The model under review builds one solid part; all positions refer to its coordinate system, in mm. Face numbers are marked on the shaded views. A direction names the side the tool comes from. Round coordinates to 2 decimals unless told otherwise and drop trailing zeros. Write each loop counter-clockwise with the first axis right and the second up, starting at its lowest first coordinate (ties: lowest second). Pieces come first, ordered by that corner, then holes. Notation, with made-up numbers: M 38,18.25 L 77,18.25 A18 cw 77,34.25 Z; hole C 28.25,-7 d2. An arc over 180 degrees is marked long. One line per item, written item: value. Start each with the question number.
1) Wall thickness on probe 1 along Y at (x, z) = (1.25, 19.5); probe 2 along Y at (x, z) = (3.5, 24); probe 3 along Z at (x, y) = (4.75, 10.5): over which ranges is each line inside the solid? List them lowest first.
2) Mouldability with a two-part tool opening along Z and no side actions: class the marked faces 1, 2 and 3 as +Z half, -Z half, draft (parallel to the pull), parting line (faces both ways), or undercut.
3) Take a section at A-A, the plane x = 5.75. Write out the cut boundary in (y, z), and give its area (3 significant figures).
4) Take a section at C-C, the plane z = 13.75. Write out the cut boundary in (x, y), and give its area (3 significant figures).
5) Tool access review of the marked faces 4, 5 and 6: name each direction out of +Z, -Z, +X, -X, +Y, -Y from which nothing blocks a thin tool from reaching the whole face with its end or side.
6) For P1, Ø1.5, axis at y = 17.5, z = 5, coming from the -X side, flat-tipped, find the tip position at first contact; note if it passes through.
7) Take a section at B-B, the plane y = 12.7. Write out the cut boundary in (x, z).
from build123d import *

# Parameters (mm, degrees)
F0_W     = 25.4
F0_H     = 25.4
F1_DEPTH = 6.35
F2_R     = 2.54
F3_DEPTH = 6.35
F4_R     = 2.54
F5_DEPTH = 6.35


with BuildPart() as f1:
    # F0 (on Right) → F1 (new body)
    with BuildSketch(Plane.YZ):
        with Locations((12.7, 12.7)):
            Rectangle(F0_W, F0_H)
    extrude(amount=F1_DEPTH)

    # F2 (on face) → F3 (cut)
    with BuildSketch(Plane.YZ.offset(6.35)):
        with Locations((12.7, 0)):
            Circle(F2_R)
        with Locations((0, 12.7)):
            Circle(F2_R)
        with Locations((12.7, 25.4)):
            Circle(F2_R)
    extrude(amount=-F3_DEPTH, mode=Mode.SUBTRACT)

    # F4 (on face) → F5 (join)
    with BuildSketch(Plane.YZ.offset(6.35)):
        with Locations((25.4, 12.7)):
            Circle(F4_R)
    extrude(amount=-F5_DEPTH)


solid = f1.part
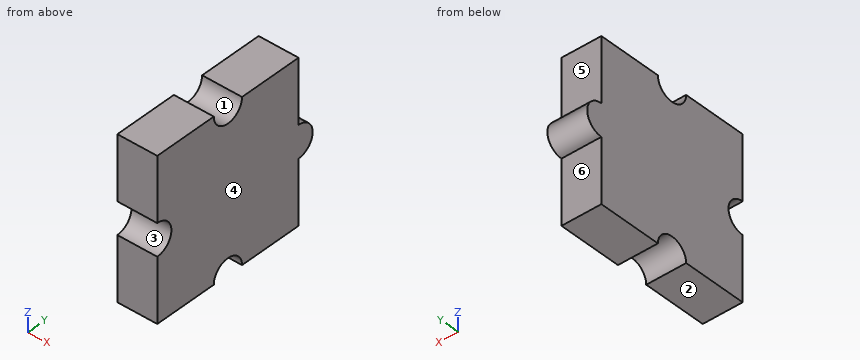
Checked values:
1. probe 1: y = 0 to 25.4
1. probe 2: y = 0 to 10.58, 14.82 to 25.4
1. probe 3: z = 1.27 to 24.13
2. face 1: +Z half
2. face 2: -Z half
2. face 3: undercut
3. outline: M 0,0 L 10.16,0 A2.54 cw 15.24,0 L 25.4,0 L 25.4,10.16 A2.54 ccw 25.4,15.24 L 25.4,25.4 L 15.24,25.4 A2.54 cw 10.16,25.4 L 0,25.4 L 0,15.24 A2.54 cw 0,10.16 Z
3. area: 625 mm2
4. outline: M 0,2.31 L 6.35,2.31 L 6.35,27.71 L 0,27.71 Z
4. area: 161 mm2
5. face 4: +Z, -Z, +X, +Y, -Y
5. face 5: +Z, +X, -X, +Y
5. face 6: -Z, +X, -X, +Y
6. P1: stops at x = 0
7. outline: M 0,2.54 L 6.35,2.54 L 6.35,22.86 L 0,22.86 Z
